```python
from build123d import *

# Parameters (mm, degrees)
SKETCH1_R                                         = 12.5
BOSS_EXTRUDE1_DEPTH                               = 5
SKETCH4_R                                         = 10
CUT_EXTRUDE1_DEPTH                                = 20
CUT_EXTRUDE2_START                                = -16.25
CUT_EXTRUDE2_DEPTH                                = 5
CSK_FOR_2_FLAT_HEAD_MACHINE_SCREW_100_D           = 2.4384
CSK_FOR_2_FLAT_HEAD_MACHINE_SCREW_100_CSINK_D     = 4.3688
CSK_FOR_2_FLAT_HEAD_MACHINE_SCREW_100_CSINK_ANGLE = 100


with BuildPart() as part:
    # Sketch1 → Boss-Extrude1 (new body)
    with BuildSketch(Plane.XY):
        Circle(SKETCH1_R)
    extrude(amount=BOSS_EXTRUDE1_DEPTH)

    # Sweep1: sweep along a curve in space
    with BuildLine() as sweep1_path:
        ThreePointArc((12.5, 0, 5), (8.838834765, 8.838834765, 5), (0, 12.5, 5))
        ThreePointArc((0, 12.5, 5), (-8.838834765, 8.838834765, 5), (-12.5, 0, 5))
        ThreePointArc((-12.5, 0, 5), (-8.838834765, -8.838834765, 5), (0, -12.5, 5))
        ThreePointArc((0, -12.5, 5), (8.838834765, -8.838834765, 5), (12.5, 0, 5))
    # Sketch3 → Sweep1 (sweep)
    with BuildSketch(Plane(origin=(0, 0, 0), x_dir=(1, 0, 0), z_dir=(0, 1, 0))):
        Polygon((0, -5), (-20, -5), (-15, -25), (0, -25), align=None)
    sweep(path=sweep1_path.line)

    # Sketch4 → Cut-Extrude1 (cut)
    with BuildSketch(Plane.XY.offset(25)):
        Circle(SKETCH4_R)
    extrude(amount=-CUT_EXTRUDE1_DEPTH, mode=Mode.SUBTRACT)

    # Sketch11 → Cut-Extrude2 (cut)
    with BuildSketch(Plane(origin=(0, 0, 0), x_dir=(1, 0, 0), z_dir=(0, 1, 0)).offset(CUT_EXTRUDE2_START)):
        with BuildLine():
            Line((-3, -10), (3, -10))
            Line((3, -10), (3, -14))
            ThreePointArc((3, -14), (0, -17), (-3, -14))
            Line((-3, -14), (-3, -10))
        make_face()
    extrude(amount=-CUT_EXTRUDE2_DEPTH, mode=Mode.SUBTRACT)

    # CSK for #2 Flat Head Machine Screw (100)2 (through all)
    with Locations(Plane(origin=(0, -16.25, 14.023346871), x_dir=(0, 0, -1), z_dir=(0, -1, 0))):
        with Locations((0, 0)):
            CounterSinkHole(CSK_FOR_2_FLAT_HEAD_MACHINE_SCREW_100_D / 2, CSK_FOR_2_FLAT_HEAD_MACHINE_SCREW_100_CSINK_D / 2, counter_sink_angle=CSK_FOR_2_FLAT_HEAD_MACHINE_SCREW_100_CSINK_ANGLE)


solid = part.part
```
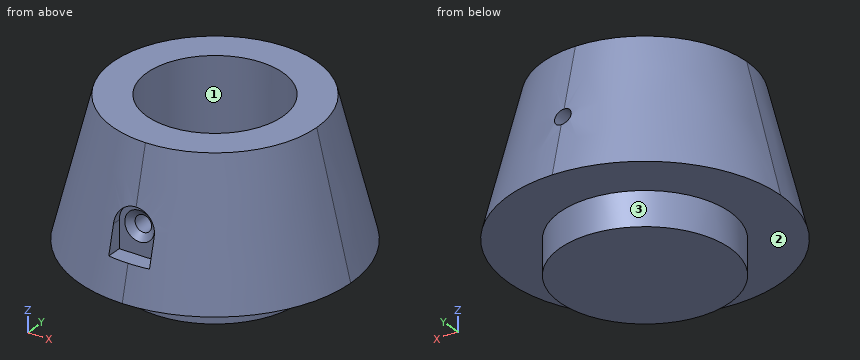
The model under review builds one solid part; all positions refer to its coordinate system, in mm. Face numbers are marked on the shaded views. Round coordinates to 2 decimals unless told otherwise and drop trailing zeros. Loops run counter-clockwise (first coordinate to the right, second up) from the corner with the lowest first, then second, coordinate; pieces in that order, holes last. Notation, with made-up numbers: (57.5, 62.5) -> (75.5, 62.5) arc R5 ccw to (75.5, 70.5) -> close; hole circle Ø10 at (78.25, 72). An arc over 180 degrees is marked (long way). Answer in a Markdown table with one row per item.
1) Consider section A-A, the plane z = 4. Write out the cut boundary in (x, y), plus the area to 3 significant figures.
Taken from the geometry:
| item | result |
|---|---|
| outline | circle Ø25 at (0, 0) |
| area | 491 mm² |
2) Consider section C-C, the plane z = 9.25. Write out the cut boundary in (x, y) (1 decimal).
Taken from the geometry:
| item | result |
|---|---|
| outline | circle Ø37.9 at (0, 0); hole circle Ø20 at (0, 0) |
3) Draft analysis for pull direction Y (two halves, no side actions). For the marked faces 1, 2 and 3, state which applies: pulls with the +Y half, pulls with the -Y half, needs draft (parallel to the pull), parting line crosses it, or undercut.
Taken from the geometry:
| item | result |
|---|---|
| face 1 | undercut |
| face 2 | needs draft |
| face 3 | parting line crosses it |
4) For pin 1 Ø10 at (y, z) = (6, 6) entering from +X; pin 2 Ø1.8 at (y, z) = (-17.5, 12) entering from -X; pin 3 Ø1.8 at (x, z) = (-1.5, 12) entering from -Y, all flat-tipped, find the tip position at first contact; note any pin that passes through.
Taken from the geometry:
| item | result |
|---|---|
| pin 1 | stops at x = 19.97 |
| pin 2 | stops at x = -7.66 |
| pin 3 | stops at y = -16.25 |
5) Consider section B-B, the plane z = 23.25. Write out the cut boundary in (x, y) (1 decimal), plus the area to 3 significant figures.
Taken from the geometry:
| item | result |
|---|---|
| outline | circle Ø30.9 at (0, 0); hole circle Ø20 at (0, 0) |
| area | 435 mm² |
6) Wall thickness on line 1 along Y through (x, z) = (-3, 7.75); line 2 along Y through (x, z) = (-3, 23.75); line 3 along Z through (x, y) = (-1, -2): over which ranges is each line inside the solid? List them lowest first.
Taken from the geometry:
| item | result |
|---|---|
| line 1 | y = -19.08 to -9.54, 9.54 to 19.08 |
| line 2 | y = -15.02 to -9.54, 9.54 to 15.02 |
| line 3 | z = 0 to 5 |
